The drawing under review shows one solid part. Ordinate dimensions are in mm from its lowest x, y, z. Give positions to 0.01 mm unless a question says otherwise; leave off trailing zeros. Loops run counter-clockwise (first coordinate to the right, second up) from the corner with the lowest first, then second, coordinate; pieces in that order, holes last. Notation, with made-up numbers: M 71.25,4 L 94.25,4 A17 ccw 94.25,17 Z; hole C 45.5,22.5 d1. An arc over 180 degrees is marked long. Write item = value, one per line. Start each with the question number.
1. We need section A-A on z = 6.35. Give the boundary of the cut face in (x, y).
2. We need section C-C on x = 19.05. Give the boundary of the cut face in (y, z).
3. We need section D-D on y = 1.1. Count the separate pieces of the cut face and the enclosed holes in it, then the cut area to 3 significant figures.
4. We need section B-B on x = 31.75. Give the boundary of the cut face in (y, z).
5. For pin 1 (0.8 mm diameter, centred on y = 0.5, z = 53.5, fed in from +X), flat-tipped, find the tip position at first contact; note if it passes through.
6. Wall thickness on line 1 along X through (y, z) = (0.55, 6.35); line 2 along Z through (x, y) = (6.35, 0.8); line 3 along Z through (x, y) = (32, 0.9): over which ranges is each line inside the solid? List them lowest first. Write a range as from..to.
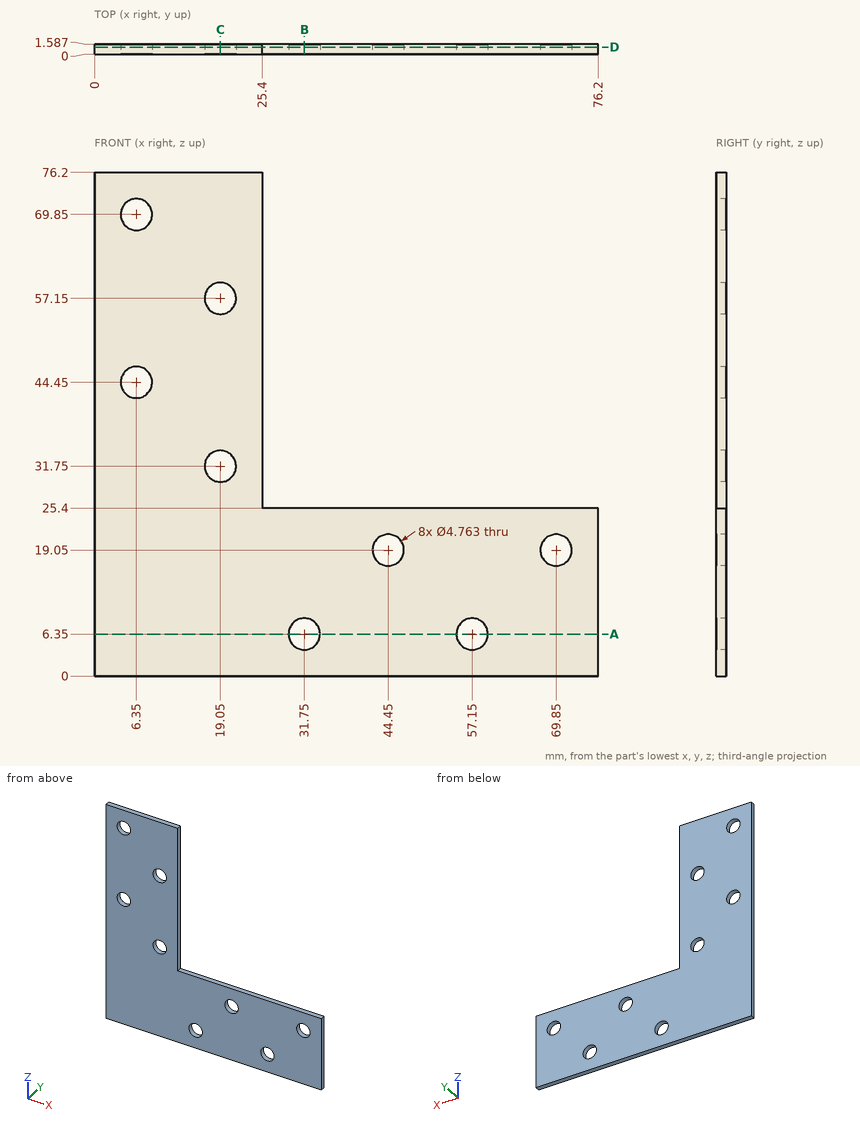
Final values:
q1.outline = M 0,0 L 29.37,0 L 29.37,1.59 L 0,1.59 Z; M 34.13,0 L 54.77,0 L 54.77,1.59 L 34.13,1.59 Z; M 59.53,0 L 76.2,0 L 76.2,1.59 L 59.53,1.59 Z
q2.outline = M 0,0 L 1.59,0 L 1.59,29.37 L 0,29.37 Z; M 0,34.13 L 1.59,34.13 L 1.59,54.77 L 0,54.77 Z; M 0,59.53 L 1.59,59.53 L 1.59,76.2 L 0,76.2 Z
q3.separate_pieces = 1
q3.enclosed_holes = 8
q3.area = 3,080 mm²
q4.outline = M 0,0 L 1.59,0 L 1.59,3.97 L 0,3.97 Z; M 0,8.73 L 1.59,8.73 L 1.59,25.4 L 0,25.4 Z
q5.pin_1 = 25.4
q6.line_1 = 0..29.37, 34.13..54.77, 59.53..76.2
q6.line_2 = 0..42.07, 46.83..67.47, 72.23..76.2
q6.line_3 = 0..3.98, 8.72..25.4
